Design review of the part built by this model. Coordinates are the model's own, in mm. Round coordinates to 2 decimals unless told otherwise and drop trailing zeros. Loops run counter-clockwise (first coordinate to the right, second up) from the corner with the lowest first, then second, coordinate; pieces in that order, holes last. Notation, with made-up numbers: M 20,79.25 L 54,79.25 A24 ccw 54,117.25 Z; hole C 67,45.25 d11. An arc over 180 degrees is marked long. One line per item, written item: value. Start each with the question number.
Item 1: Clearance check with flat-ended pins moving along their axes: pin 1 (3 mm diameter, centred on x = 35, y = -63.5, fed in from +Z); pin 2 (2.5 mm diameter, centred on x = -28, y = -49, fed in from +Z). State where each tip first meets the part, or that it passes through.
Item 2: Mouldability with a two-part tool opening along Y and no side actions: class faces 1 (the flat face through (32.05, -45, 22)), 2 (the flat face through (7, 0, 2)) as released by +Y, released by -Y, zero draft, split by the parting line, or undercut.
Item 3: We need section D-D (x = 28). Write out the cut boundary in (y, z).
Item 4: For line 1 along Z through (x, y) = (20.5, -31); line 2 along Z through (x, y) = (5.5, -28.5), list the stretches that pass through material, from the lowest coordinate up.
Item 5: We need section B-B (x = -8). Write out the cut boundary in (y, z).
Item 6: We need section A-A (z = 35.5). State how many separate pieces and enclosed holes the cut face has, then the cut area to 3 significant figures.
from build123d import *

# Parameters (mm, degrees)
PAD_DEPTH = 90.5


with BuildPart() as part:
    # Sketch → Pad (new body)
    with BuildSketch(Plane.XZ):
        Polygon((-45.25, 0), (-45.25, 40), (-43.65, 40), (-43.65, 4.2), (-39.35, 4.2), (-39.35, 40), (-37.85, 40), (-37.85, 4.2), (-32.05, 4.2), (-32.05, 40), (-30.55, 40), (-30.55, 9.8), (-25.55, 9.8), (-25.309162, 40), (-24.109162, 40), (-23.868323, 9.8), (-18.868323, 9.8), (-18.627485, 40), (-17.427485, 40), (-17.141988, 4.2), (-12.141988, 4.2), (-11.856491, 40), (-10.656491, 40), (-10.370994, 4.2), (-5.370994, 4.2), (-5.085497, 40), (-3.885497, 40), (-3.6, 4.2), (3.6, 4.2), (3.885497, 40), (5.085497, 40), (5.370994, 4.2), (10.370994, 4.2), (10.656491, 40), (11.856491, 40), (12.141988, 4.2), (17.141988, 4.2), (17.427485, 40), (18.627485, 40), (18.868323, 9.8), (23.868323, 9.8), (24.109162, 40), (25.309162, 40), (25.55, 9.8), (30.55, 9.8), (30.55, 40), (32.05, 40), (32.05, 4.2), (37.85, 4.2), (37.85, 40), (39.35, 40), (39.35, 4.2), (43.65, 4.2), (43.65, 40), (45.25, 40), (45.25, 0), align=None)
    extrude(amount=PAD_DEPTH)


solid = part.part
A:
1. pin 1: z = 4.2
1. pin 2: z = 9.8
2. face 1: zero draft
2. face 2: released by +Y
3. outline: M -90.5,0 L 0,0 L 0,9.8 L -90.5,9.8 Z
4. line 1: 0 to 9.8
4. line 2: 0 to 4.2
5. outline: M -90.5,0 L 0,0 L 0,4.2 L -90.5,4.2 Z
6. separate pieces: 14
6. enclosed holes: 0
6. area: 1,750 mm2
